Here's how the part is built. I have some questions about the finished solid (model axes, mm). Face numbers are marked on the shaded views. A direction names the side the tool comes from. Round coordinates to 2 decimals unless told otherwise and drop trailing zeros. Loops run counter-clockwise (first coordinate to the right, second up) from the corner with the lowest first, then second, coordinate; pieces in that order, holes last. Notation, with made-up numbers: M 75.5,31 L 98.5,31 A19 cw 98.5,47 Z; hole C 30.25,60.25 d8. An arc over 180 degrees is marked long. Use a Markdown table: item, result.
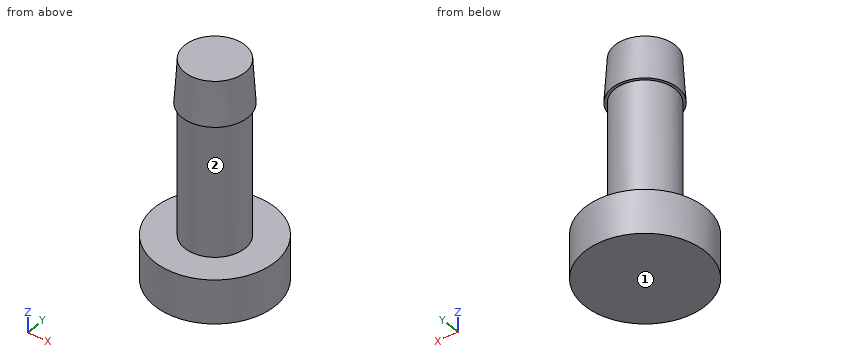
```python
from build123d import *

# Parameters (mm, degrees)
F0_R      = 2.75
F0_R_2    = 1.375
F1_DEPTH  = 2
F2_DEPTH  = 10
F4_R      = 1.5
F2_FACE_R = 1.375


with BuildPart() as f1:
    # F0 (on Top) → F1 (new body)
    with BuildSketch(Plane.XY):
        Circle(F0_R)
        Circle(F0_R_2, mode=Mode.SUBTRACT)
        Circle(F0_R_2)
    extrude(amount=F1_DEPTH)

    # F0 (on Top) → F2 (join)
    with BuildSketch(Plane.XY):
        Circle(F0_R_2)
    extrude(amount=F2_DEPTH)

    # F4 (on offset) → F5 section 0
    with BuildSketch(Plane.XY.offset(8)):
        Circle(F4_R)
    # F2_face (on face) → F5 section 1
    with BuildSketch(Plane.XY.offset(10)):
        Circle(F2_FACE_R)
    loft()


solid = f1.part
```
Q1. Imagine slicing it at A-A, the plane x = 0. Please give me the cut outline in (y, z) (3 decimals).
Return value:
| item | result |
|---|---|
| outline | M -2.75,0 L 2.75,0 L 2.75,2 L 1.375,2 L 1.375,8 L 1.5,8 L 1.375,10 L -1.375,10 L -1.5,8 L -1.375,8 L -1.375,2 L -2.75,2 Z |
Q2. Imagine slicing it at C-C, the plane y = 1.65. Please give me the cut outline in (x, z).
Return value:
| item | result |
|---|---|
| outline | M -2.2,0 L 2.2,0 L 2.2,2 L -2.2,2 Z |
Q3. Imagine slicing it at D-D, the plane x = 2.05. Please give me the cut outline in (y, z), then the cut area to 3 significant figures.
Return value:
| item | result |
|---|---|
| outline | M -1.83,0 L 1.83,0 L 1.83,2 L -1.83,2 Z |
| area | 7.33 mm^2 |
Q4. Imagine slicing it at B-B, the plane z = 6.5. Please give me the cut outline in (x, y) (3 decimals), then the cut area to 3 significant figures.
Return value:
| item | result |
|---|---|
| outline | C 0,0 d2.75 |
| area | 5.94 mm^2 |
Q5. I need wall thicknesses on line 1 (Z direction, x = 2.4, y = 0.45); line 2 (X direction, y = 2.05, z = 0.75); line 3 (X direction, y = -0.75, z = 6). Which ranges of each line are inside material? Lowest first, please. Write a range as from..to.
Return value:
| item | result |
|---|---|
| line 1 | z = 0..2 |
| line 2 | x = -1.83..1.83 |
| line 3 | x = -1.15..1.15 |
Q6. For the marked faces 1 and 2, which set-ups out of +Z, -Z, +X, -X, +Y, -Y let a thin tool reach every point of the face, with its end or its side?
Return value:
| item | result |
|---|---|
| face 1 | -Z, +X, -X, +Y, -Y |
| face 2 | none |
